The listing builds one solid part. Answer for the finished solid, in the listing's coordinates (mm). Coordinates: 2 decimals unless noted, no trailing zeros. Order: outer loops, then holes, each group sorted by start corner. A loop starts at its lowest first (then second) coordinate and runs counter-clockwise, first axis right, second up. Notation, with made-up numbers: (73, -20) -> (78, -20) arc R15 ccw to (78, 8) -> close; hole circle Ø8 at (-37.75, 77.25). An arc over 180 degrees is marked (long way). Write item = value, one per line. Start each with the question number.
```python
from build123d import *

# Parameters (mm, degrees)
PAD_DEPTH = 10


with BuildPart() as part:
    # Sketch → Pad (new body)
    with BuildSketch(Plane.XY):
        with BuildLine():
            ThreePointArc((30.793243, 28.920895), (6.376554, 23.603742), (30.12088, 15.815685))
            Line((30.12088, 15.815685), (40.865706, 12.784345))
            Line((40.865706, 12.784345), (47.180485, 21.991074))
            Line((47.180485, 21.991074), (41.614066, 31.668641))
            Line((41.614066, 31.668641), (30.793243, 28.920895))
        make_face()
    extrude(amount=PAD_DEPTH)


solid = part.part
```
Item 1: Section A-A, the plane z = 4.5 is taken. Give the vertices of the cut face in (x, y).
Item 2: For a pull along X with two mould halves and no side action, classify faces 1 (the flat face through (35.42, 14.32, 4.93)), 2 (the flat face through (26, 23, 0)), 3 (the flat face through (43.979, 17.323, 4.93)), 4 (the flat face through (36.279, 30.314, 4.93)) as pulls with the +X half, pulls with the -X half, needs draft (parallel to the pull), parting line crosses it, or undercut.
Item 3: Section D-D, the plane x = 26.5 is taken. Give the vertices of the cut face in (y, z), then the cut area to 3 significant figures.
Item 4: Section B-B, the plane y = 15.25 is taken. Give the vertices of the cut face in (x, z), then the cut area to 3 significant figures.
Item 5: Consider probe 1 along Y at (x, z) = (35, 2.75); probe 2 along X at (y, z) = (28.5, 6.75); probe 3 along X at (y, z) = (33.25, 7). Determine where each line is inside the solid, lowest interval first.
Item 6: Each of these flat-tipped pins is pushed along its axis until it touches: pin 1 (5 mm diameter, centred on y = 31.5, z = 2.5, fed in from -X); pin 2 (5 mm diameter, centred on x = 29, z = 8, fed in from +Y). Where does it stop, or does it pass through?
Item 7: Section C-C, the plane y = 29.75 is taken. Give the vertices of the cut face in (x, z), then the cut area to 3 significant figures.
A:
q1.outline = (30.12, 15.82) -> (40.87, 12.78) -> (47.18, 21.99) -> (41.61, 31.67) -> (30.79, 28.92) arc R12.95 ccw (long way) to start
q2.face_1 = undercut
q2.face_2 = needs draft
q2.face_3 = pulls with the +X half
q2.face_4 = undercut
q3.outline = (12.17, 0) -> (33.71, 0) -> (33.71, 10) -> (12.17, 10) -> close
q3.area = 215 mm^2
q4.outline = (8.89, 0) -> (29.73, 0) -> (29.73, 10) -> (8.89, 10) -> close; (32.13, 0) -> (42.56, 0) -> (42.56, 10) -> (32.13, 10) -> close
q4.area = 313 mm^2
q5.probe_1 = 14.44 to 29.99
q5.probe_2 = 7.61 to 43.44
q5.probe_3 = 11.47 to 27.14
q6.pin_1 = 7.86
q6.pin_2 = 33.71
q7.outline = (8.29, 0) -> (30.32, 0) -> (30.32, 10) -> (8.29, 10) -> close; (34.06, 0) -> (42.72, 0) -> (42.72, 10) -> (34.06, 10) -> close
q7.area = 307 mm^2
